Read the model definition and answer for the solid it produces. Units are mm, in the model's axes. Face numbers are marked on the shaded views. Give positions to 0.01 mm unless a question says otherwise; leave off trailing zeros. Write each loop counter-clockwise with the first axis right and the second up, starting at its lowest first coordinate (ties: lowest second). Pieces come first, ordered by that corner, then holes. Notation, with made-up numbers: (15, 40) -> (51, 40) arc R37 cw to (51, 79) -> close; hole circle Ø9 at (-6.5, -19.75). An arc over 180 degrees is marked (long way). Use a Markdown table: item, result.
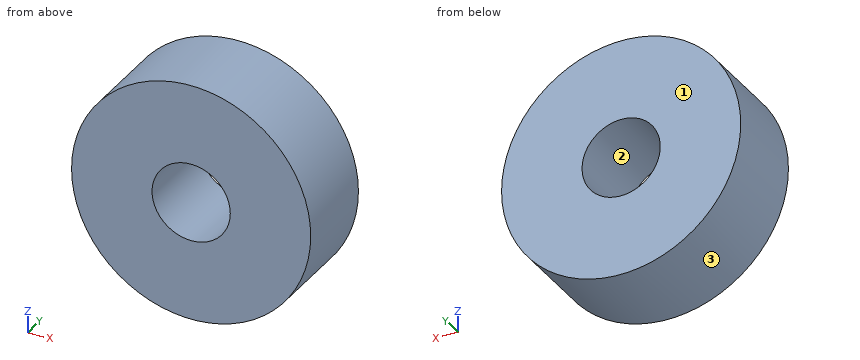
from build123d import *

# Parameters (mm, degrees)
CYLINDER015_R            = 0.9
CYLINDER015_DEPTH        = 2
CYLINDER014_R            = 2.75
CYLINDER014_DEPTH        = 2
CLONE016_PLACEMENT_ANGLE = 90


with BuildPart() as faceanchorscrewhole:
    # Cylinder015 → Cylinder015 (new body)
    with BuildSketch(Plane.XY):
        Circle(CYLINDER015_R)
    extrude(amount=CYLINDER015_DEPTH)


with BuildPart() as faceanchor002:
    # Cylinder014 → Cylinder014 (new body)
    with BuildSketch(Plane.XY):
        Circle(CYLINDER014_R)
    extrude(amount=CYLINDER014_DEPTH)

    # Cut015: cut FaceAnchorScrewHole
    add(faceanchorscrewhole.part, mode=Mode.SUBTRACT)


with BuildPart() as faceanchor002_1:
    # Clone016 placement: moved
    add(faceanchor002.part.moved(Location((110, 2, 35))).rotate(Axis((110, 2, 35), (1, 0, 0)), CLONE016_PLACEMENT_ANGLE))


solid = faceanchor002_1.part
Item 1: Straight lines are drawn through the part: line 1 along Z through (x, y) = (110, 1.45); line 2 along X through (y, z) = (1.6, 34.85); line 3 along X through (y, z) = (1.8, 34.7). For each, find the intervals that lie inside material, in ascending order. Write a range as [from, to].
Return value:
| item | result |
|---|---|
| line 1 | [32.25, 34.1], [35.9, 37.75] |
| line 2 | [107.25, 109.11], [110.89, 112.75] |
| line 3 | [107.27, 109.15], [110.85, 112.73] |
Item 2: A cutting plane is placed at B-B (z = 35). Give the vertices of the cut face in (x, y).
Return value:
| item | result |
|---|---|
| outline | (107.25, 0) -> (109.1, 0) -> (109.1, 2) -> (107.25, 2) -> close; (110.9, 0) -> (112.75, 0) -> (112.75, 2) -> (110.9, 2) -> close |
Item 3: A cutting plane is placed at D-D (x = 111.7). Give the vertices of the cut face in (y, z), then the cut area to 3 significant figures.
Return value:
| item | result |
|---|---|
| outline | (0, 32.84) -> (2, 32.84) -> (2, 37.16) -> (0, 37.16) -> close |
| area | 8.65 mm^2 |
Item 4: For a pull along Z with two mould halves and no side action, classify the marked faces 1, 2 and 3 as +Z half, -Z half, draft (parallel to the pull), parting line (faces both ways), or undercut.
Return value:
| item | result |
|---|---|
| face 1 | draft |
| face 2 | undercut |
| face 3 | parting line |
Item 5: A cutting plane is placed at C-C (y = 1.85). Give the vertices of the cut face in (x, z), then the cut area to 3 significant figures.
Return value:
| item | result |
|---|---|
| outline | circle Ø5.5 at (110, 35); hole circle Ø1.8 at (110, 35) |
| area | 21.2 mm^2 |
Item 6: A cutting plane is placed at A-A (x = 110). Give the vertices of the cut face in (y, z).
Return value:
| item | result |
|---|---|
| outline | (0, 32.25) -> (2, 32.25) -> (2, 34.1) -> (0, 34.1) -> close; (0, 35.9) -> (2, 35.9) -> (2, 37.75) -> (0, 37.75) -> close |
Item 7: This flat-tipped pin is pushed along its axis until it touches: P1, Ø3, axis at x = 110, z = 35, coming from the -Y side. Where does it stop, or does it pass through?
Return value:
| item | result |
|---|---|
| P1 | y = 0 |
